Verification items for the finished model (mm, model axes). Give positions to 0.01 mm unless a question says otherwise; leave off trailing zeros. Loops run counter-clockwise (first coordinate to the right, second up) from the corner with the lowest first, then second, coordinate; pieces in that order, holes last. Notation, with made-up numbers: (-26.5, 44.5) - (11.5, 44.5) arc R22 cw to (11.5, 57.5) - close; hole circle Ø6 at (-17, 47). An arc over 180 degrees is marked (long way). One line per question, with ' | ' between items. Start each with the question number.
1. Section check B-B, the plane y = 0. Enter the section's corners in (x, z).
2. Mould release check, pull along Y, two halves, no side actions. Record for faces 1 (the face through (-9, 0, 5)), 2 (the face through (8.43, 8.4, 5.07)), 3 (the face through (-6, 0, 5)): +Y half, -Y half, draft (parallel to the pull), parting line (faces both ways), or undercut.
3. Thickness scan on line 1 along Y through (x, z) = (0, 5.75); line 2 along Y through (x, z) = (-4.75, 6.5); line 3 along X through (y, z) = (2, 4). Record the ranges inside material, lowest first. Write a range as from..to.
4. Section check A-A, the plane z = 4.75. Enter the section's corners in (x, y), then the cut area to 3 significant figures.
5. Section check D-D, the plane x = -8. Enter the section's corners in (y, z), then the cut area to 3 significant figures.
Autodesk Inventor part; units mm, degrees
ref_plane "YZ Plane" through (0, 0, 0) normal (1, 0, 0) x (0, 1, 0)
ref_plane "XZ Plane" through (0, 0, 0) normal (0, 1, 0) x (-1, 0, 0)
ref_plane "XY Plane" through (0, 0, 0) normal (0, 0, 1) x (1, 0, 0)
sketch "Skizze1" plane through (0, 0, 0) normal (0, 0, 1) x (1, 0, 0)
  line L0 (9, -9) -> (-9, -9)
  line L1 (-9, -9) -> (-9, 9)
  line L2 (-9, 9) -> (9, 9)
  line L3 (9, 9) -> (9, -9)
  line L4 (9, -9) -> (-9, 9) construction
  line L5 (-9, -9) -> (9, 9) construction
  circle A0 centre (0, 0) radius 6
  dimension "d0" = 18
  dimension "d1" = 18
  dimension "d2" = 12
extrude "Extrusion1" add sketch "Skizze1" along normal blind 10
fillet "Rundung1" radius 2 4 edges at (9, 9, 5) (-9, 9, 5) (9, -9, 5) (-9, -9, 5)
properties part number "00_CCTV_M12_VCM"
Results list:
1) outline: (-9, 0) - (-6, 0) - (-6, 10) - (-9, 10) - close; (6, 0) - (9, 0) - (9, 10) - (6, 10) - close
2) face 1: draft | face 2: +Y half | face 3: undercut
3) line 1: -9..-6, 6..9 | line 2: -9..-3.67, 3.67..9 | line 3: -9..-5.66, 5.66..9
4) outline: (-9, -7) arc R2 ccw to (-7, -9) - (7, -9) arc R2 ccw to (9, -7) - (9, 7) arc R2 ccw to (7, 9) - (-7, 9) arc R2 ccw to (-9, 7) - close; hole circle Ø12 at (0, 0) | area: 207 mm²
5) outline: (-8.73, 0) - (8.73, 0) - (8.73, 10) - (-8.73, 10) - close | area: 175 mm²
